from build123d import *

# Parameters (mm, degrees)
BOSS_EXTRUDE1_DEPTH = 10
SKETCH2_R           = 3
CUT_EXTRUDE1_DEPTH  = 27
SKETCH4_R           = 19.5
SKETCH4_R_2         = 13
BOSS_EXTRUDE2_DEPTH = 3
CUT_EXTRUDE2_DEPTH  = 8
CHAMFER1_SIZE       = 3
SKETCH6_W           = 41.436134758
SKETCH6_H           = 7.128250764
CUT_EXTRUDE3_DEPTH  = 5
FILLET1_R           = 3.65


# Some blends are built 0.0001 mm under size
with BuildPart() as part:
    # Sketch1 → Boss-Extrude1 (new body)
    with BuildSketch(Plane(origin=(0, 0, 0), x_dir=(1, 0, 0), z_dir=(0, 1, 0))):
        with BuildLine():
            Line((-16.306566162, -4), (-31.007810594, -4))
            Line((-31.007810594, -4), (-31.007810594, -29))
            Line((-31.007810594, -29), (-22, -29))
            Line((-22, -29), (22, -29))
            Line((22, -29), (31.007810594, -29))
            Line((31.007810594, -29), (31.007810594, -4))
            Line((31.007810594, -4), (16.306566162, -4))
            ThreePointArc((16.306566162, -4), (0, -16.79), (-16.306566162, -4))
        make_face()
    extrude(amount=BOSS_EXTRUDE1_DEPTH)

    # Sketch2 → Cut-Extrude1 (cut)
    with BuildSketch(Plane(origin=(0, 0, 4), x_dir=(-1, 0, 0), z_dir=(0, 0, -1))):
        with Locations((-26.007810594, 5)):
            Circle(SKETCH2_R)
        with Locations((26.007810594, 5)):
            Circle(SKETCH2_R)
    extrude(amount=-CUT_EXTRUDE1_DEPTH, mode=Mode.SUBTRACT)

    # Sketch4 → Boss-Extrude2 (add)
    with BuildSketch(Plane(origin=(0, 10, 0), x_dir=(1, 0, 0), z_dir=(0, 1, 0))):
        with Locations(Location((0, 0, 0), (0, 0, 348.162995844))):
            Circle(SKETCH4_R)
        with Locations(Location((0, 0, 0), (0, 0, 270))):
            Circle(SKETCH4_R_2, mode=Mode.SUBTRACT)
    extrude(amount=BOSS_EXTRUDE2_DEPTH)

    # Sketch5 → Cut-Extrude2 (cut)
    with BuildSketch(Plane(origin=(0, 13, 0), x_dir=(1, 0, 0), z_dir=(0, 1, 0))):
        Polygon((-19.085334684, -4), (-23.625672229, -4), (-23.625672229, 24.113520256), (25.409917146, 24.113520256), (25.409917146, -4), align=None)
    extrude(amount=-CUT_EXTRUDE2_DEPTH, mode=Mode.SUBTRACT)

    # Chamfer1
    chamfer1_edges = [part.edges().sort_by_distance(p)[0] for p in [
        (0, 10, 19.5),
    ]]
    chamfer(chamfer1_edges, length=CHAMFER1_SIZE - 0.0001)  # a hair under: the kernel refuses the full size

    # Sketch6 → Cut-Extrude3 (cut)
    with BuildSketch(Plane.XZ):
        with Locations((0, 22.895)):
            Rectangle(SKETCH6_W, SKETCH6_H)
    extrude(amount=-CUT_EXTRUDE3_DEPTH, mode=Mode.SUBTRACT)

    # Fillet1
    # the kernel refuses this fillet: 3.65 mm, written as the material it adds along each edge
    with BuildSketch(Plane(origin=(-20.718067379, 0, 19.330874618), x_dir=(0, 0, 1), z_dir=(0, 1, 0))) as fillet1_piece_1:
        with BuildLine():
            CenterArc((FILLET1_R, FILLET1_R), FILLET1_R, 180, 90)
            Line((0, FILLET1_R), (0, 0))
            Line((0, 0), (FILLET1_R, 0))
        make_face()
    extrude(amount=5)
    with BuildSketch(Plane(origin=(-20.718067379, 0, 26.459125382), x_dir=(0, 0, -1), z_dir=(0, 1, 0)), Plane(origin=(20.718067379, 0, 26.459125382), x_dir=(-1, 0, 0), z_dir=(0, 1, 0)), Plane(origin=(20.718067379, 0, 19.330874618), x_dir=(0, 0, 1), z_dir=(0, 1, 0))) as fillet1_piece_2:
        with BuildLine():
            CenterArc((FILLET1_R, -FILLET1_R), FILLET1_R, 90, 90)
            Line((0, -FILLET1_R), (0, 0))
            Line((0, 0), (FILLET1_R, 0))
        make_face()
    extrude(amount=5)


solid = part.part
Verification items for the finished model (mm, model axes). A direction names the side the tool comes from. Coordinates: 2 decimals unless noted, no trailing zeros. Write each loop counter-clockwise with the first axis right and the second up, starting at its lowest first coordinate (ties: lowest second). Pieces come first, ordered by that corner, then holes. Notation, with made-up numbers: M 50,-28.5 L 106,-28.5 A17 cw 106,0.5 Z; hole C 26.5,0 d7. An arc over 180 degrees is marked long. Use a Markdown table: item, result.
Q1. Sectioned sample at C-C, the plane y = 7. Record the boundary of the cut face in (x, z).
Reply:
| item | result |
|---|---|
| outline | M -31.01,4 L -28.24,4 L -28.24,29 L -31.01,29 Z; M -23.77,4 L -16.31,4 A16.79 cw 16.31,4 L 23.77,4 L 23.77,29 L -23.77,29 Z; M 28.24,4 L 31.01,4 L 31.01,29 L 28.24,29 Z |
Q2. Draft check along Z on faces 1 (the face through (0, 2, 26.459)), 2 (the face through (-28.8, 3.9, 16.3)), 3 (the face through (22, 7, 4)). Enter one of: +Z half, -Z half, draft (parallel to the pull), parting line (faces both ways), or undercut.
Reply:
| item | result |
|---|---|
| face 1 | undercut |
| face 2 | draft |
| face 3 | -Z half |
Q3. Sectioned sample at D-D, the plane z = 14.25. Count the separate pieces of the cut face and the enclosed holes in it, plus the area to 3 significant figures.
Reply:
| item | result |
|---|---|
| separate pieces | 1 |
| enclosed holes | 2 |
| area | 478 mm² |
Q4. Thickness scan on line 1 (X direction, y = 5, z = 13); line 2 (X direction, y = 4, z = 13.25); line 3 (Y direction, x = 14, z = 19.25). Record the ranges inside material, lowest first.
Reply:
| item | result |
|---|---|
| line 1 | x = -31.01 to -29.01, -23.01 to -10.63, 10.63 to 23.01, 29.01 to 31.01 |
| line 2 | x = -31.01 to -28.84, -23.18 to -10.31, 10.31 to 23.18, 28.84 to 31.01 |
| line 3 | y = 0 to 10 |
Q5. Sectioned sample at B-B, the plane x = 27. Record the boundary of the cut face in (y, z).
Reply:
| item | result |
|---|---|
| outline | M 0,4 L 2.17,4 L 2.17,29 L 0,29 Z; M 7.83,4 L 10,4 L 10,29 L 7.83,29 Z |
Q6. Go/stop test with flat-tipped pins: P1, Ø1, axis at x = 6, z = 15, coming from the -Y side; P2, Ø5.5, axis at x = -1.5, y = 3.5, coming from the -Z side; P3, Ø5, axis at x = 22, z = 8, coming from the +Y side. Record where each tip stops, or that it passes through.
Reply:
| item | result |
|---|---|
| P1 | stops at y = 10 |
| P2 | stops at z = 16.24 |
| P3 | stops at y = 11.59 |
Q7. Sectioned sample at A-A, the plane y = 3.5. Record the boundary of the cut face in (x, z) (3 decimals), plus the area to 3 significant figures.
Reply:
| item | result |
|---|---|
| outline | M -31.008,4 L -28.606,4 L -28.606,29 L -31.008,29 Z; M -23.41,4 L -16.307,4 A16.79 cw 16.307,4 L 23.41,4 L 23.41,29 L -23.41,29 Z; M 28.606,4 L 31.008,4 L 31.008,29 L 28.606,29 Z; hole M -20.717,22.895 A3.65 ccw -17.068,19.331 L 17.068,19.331 A3.65 ccw 20.717,22.895 A3.65 ccw 17.068,26.459 L -17.068,26.459 A3.65 ccw Z |
| area | 697 mm² |
Q8. Set-up check for faces 4 (the face through (0.313, 4.93, 16.787)), 5 (the face through (-19.59, 2.46, 20.34)), 6 (the face through (0, 10, 25)), 7 (the face through (-22, 7, 4)): record each of +Z, -Z, +X, -X, +Y, -Y from which the full face is reachable in a straight line by a thin tool's end or side.
Reply:
| item | result |
|---|---|
| face 4 | -Z, -Y |
| face 5 | -Y |
| face 6 | +Z, +Y |
| face 7 | -Z, +X, -X, +Y, -Y |
